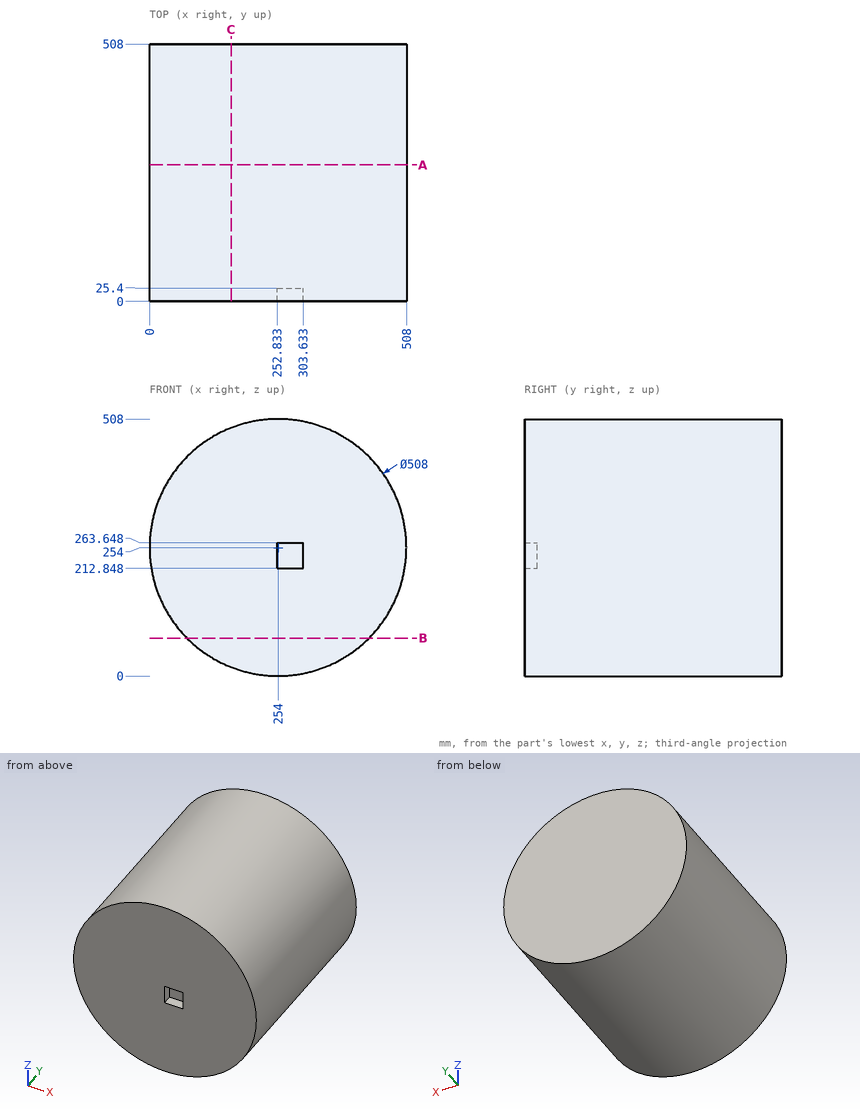
Design review of the part shown in the three views and the two pictorial views. Dimensions are in mm from the part's minimum x, y and z. Round coordinates to 2 decimals unless told otherwise and drop trailing zeros. Loops run counter-clockwise (first coordinate to the right, second up) from the corner with the lowest first, then second, coordinate; pieces in that order, holes last. Notation, with made-up numbers: (-17.75, 36) -> (35.25, 36) arc R3 cw to (35.25, 41) -> close; hole circle Ø9 at (-22, 17). An arc over 180 degrees is marked (long way). Use one line per item in the form item = value. Start each with the question number.
Q1. We need section A-A on y = 269. Give the boundary of the cut face in (x, z), then the cut area to 3 significant figures.
Q2. We need section B-B on z = 75. Give the boundary of the cut face in (x, y).
Q3. For pin 1 Ø4 at (y, z) = (372.5, 105.5) entering from +X (1 decimal); pin 2 Ø3 at (x, z) = (350, 421) entering from -Y; pin 3 Ø4 at (x, y) = (334, 75.5) entering from -Z; pin 4 Ø5 at (x, y) = (166.5, 119.5) entering from -Z (1 decimal), all flat-tipped, find the tip position at first contact; note any pin that passes through.
Q4. We need section C-C on x = 161.5. Give the boundary of the cut face in (y, z), then the cut area to 3 significant figures.
Q5. Wall thickness on line 1 along Z through (x, y) = (145, 409); line 2 along X through (y, z) = (84.5, 89.5) (1 decimal); line 3 along X through (y, z) = (34, 231.5): over which ranges is each line inside the solid? List them lowest first. Write a range as [from, to].
Calculated:
q1.outline = circle Ø508 at (254, 254)
q1.area = 203,000 mm²
q2.outline = (73.79, 0) -> (434.21, 0) -> (434.21, 508) -> (73.79, 508) -> close
q3.pin_1 = 461.5
q3.pin_2 = 0
q3.pin_3 = 12.27
q3.pin_4 = 14.6
q4.outline = (0, 17.44) -> (508, 17.44) -> (508, 490.56) -> (0, 490.56) -> close
q4.area = 240,000 mm²
q5.line_1 = [24.58, 483.42]
q5.line_2 = [60.5, 447.5]
q5.line_3 = [1, 507]
